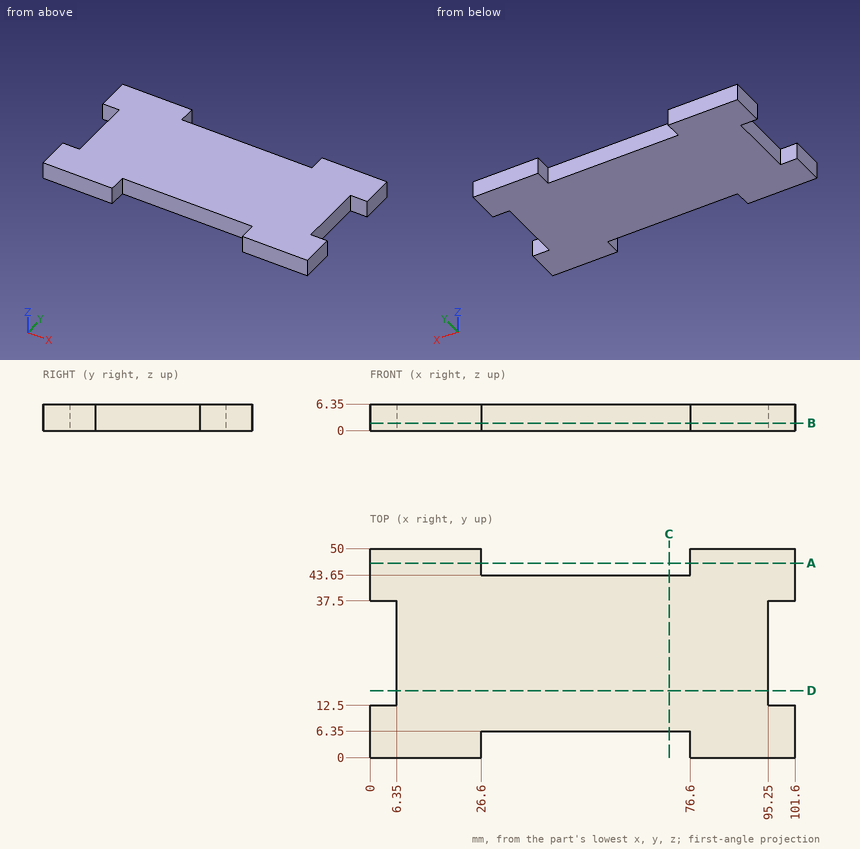
Answer from the drawing. Dimensions are ordinates in mm from the lowest x, y and z of the part. Give positions to 0.01 mm unless a question says otherwise; leave off trailing zeros. Order: outer loops, then holes, each group sorted by start corner. A loop starts at its lowest first (then second) coordinate and runs counter-clockwise, first axis right, second up. Notation, with made-up numbers: (43.25, 32) - (53.25, 32) arc R21 ccw to (53.25, 60) - close; hole circle Ø7 at (11, 34). An arc over 180 degrees is marked (long way). One line per item, written item: value. Start each with the question number.
1) Given pin 1 Ø3 at (x, y) = (54, 22) entering from -Z; pin 2 Ø3 at (y, z) = (24, 1) entering from +X; pin 3 Ø2 at (y, z) = (18, 2) entering from -X, each flat-ended and moving along its own axis, determine where each tip first touches the part or whether it passes through.
2) A cutting plane is placed at B-B on z = 1.75. Give the vertices of the cut face in (x, y), then the cut area to 3 significant figures.
3) Find the intervals of material crossed by L1, parallel to X at y = 4, z = 0.75; L2, parallel to X at y = 21, z = 3.5; L3, parallel to Y at x = 44, z = 3.25, in increasing order.
4) A cutting plane is placed at C-C on x = 71.5. Give the vertices of the cut face in (y, z), then the cut area to 3 significant figures.
5) A cutting plane is placed at D-D on y = 16. Give the vertices of the cut face in (x, z), then the cut area to 3 significant figures.
6) A cutting plane is placed at A-A on y = 46.5. Give the vertices of the cut face in (x, z).
Answer sheet:
1. pin 1: stops at z = 0
1. pin 2: stops at x = 95.25
1. pin 3: stops at x = 6.35
2. outline: (0, 0) - (26.6, 0) - (26.6, 6.35) - (76.6, 6.35) - (76.6, 0) - (101.6, 0) - (101.6, 12.5) - (95.25, 12.5) - (95.25, 37.5) - (101.6, 37.5) - (101.6, 50) - (76.6, 50) - (76.6, 43.65) - (26.6, 43.65) - (26.6, 50) - (0, 50) - (0, 37.5) - (6.35, 37.5) - (6.35, 12.5) - (0, 12.5) - close
2. area: 4,130 mm2
3. L1: x = 0 to 26.6, 76.6 to 101.6
3. L2: x = 6.35 to 95.25
3. L3: y = 6.35 to 43.65
4. outline: (6.35, 0) - (43.65, 0) - (43.65, 6.35) - (6.35, 6.35) - close
4. area: 237 mm2
5. outline: (6.35, 0) - (95.25, 0) - (95.25, 6.35) - (6.35, 6.35) - close
5. area: 565 mm2
6. outline: (0, 0) - (26.6, 0) - (26.6, 6.35) - (0, 6.35) - close; (76.6, 0) - (101.6, 0) - (101.6, 6.35) - (76.6, 6.35) - close
